For this review, take the finished solid that the model builds, in its own axes (mm). Face numbers are marked on the shaded views. A direction names the side the tool comes from. Give positions to 0.01 mm unless a question says otherwise; leave off trailing zeros. Loops run counter-clockwise (first coordinate to the right, second up) from the corner with the lowest first, then second, coordinate; pieces in that order, holes last. Notation, with made-up numbers: (85, -37) - (143, -37) arc R16 cw to (143, -32) - close; hole circle Ø2 at (5.25, 83). An arc over 180 degrees is marked (long way). Put each result on its own line as item: value. Start each with the question number.
from build123d import *

# Parameters (mm, degrees)
F0_W     = 40
F0_H     = 20
F1_DEPTH = 10
F2_DEPTH = 30
F3_DEPTH = 20
F4_W     = 10
F4_H     = 10
F5_DEPTH = 25


with BuildPart() as f1:
    # F0 (on Top) → F1 (new body)
    with BuildSketch(Plane.XY):
        Polygon((0, 40), (0, 20), (40, 20), (50, 20), (50, 40), align=None)
        with Locations((20, 10)):
            Rectangle(F0_W, F0_H)
        Polygon((40, 20), (40, 0), (60, 0), (60, 20), (50, 20), align=None)
    extrude(amount=-F1_DEPTH)

    # F0 (on Top) → F2 (join)
    with BuildSketch(Plane.XY):
        Polygon((0, 40), (0, 20), (40, 20), (50, 20), (50, 40), align=None)
    extrude(amount=F2_DEPTH)

    # F0 (on Top) → F3 (join)
    with BuildSketch(Plane.XY):
        Polygon((40, 20), (40, 0), (60, 0), (60, 20), (50, 20), align=None)
    extrude(amount=F3_DEPTH)

    # F4 (on face) → F5 (cut)
    with BuildSketch(Plane.YZ.offset(60)):
        with Locations((5, 5)):
            Rectangle(F4_W, F4_H)
    extrude(amount=-F5_DEPTH, mode=Mode.SUBTRACT)


solid = f1.part
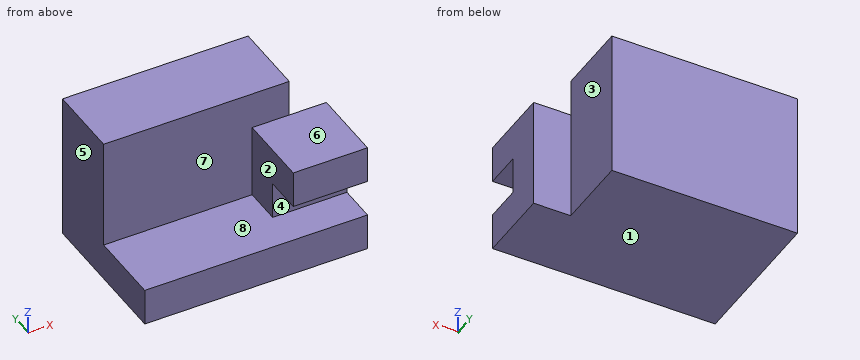
1) Machinability: for the marked faces 1, 2, 3, 4 and 5, which of the approach directions +Z, -Z, +X, -X, +Y, -Y give a long, thin tool a straight path to every point of the face, cutting with its end or side? Answer none if there is none.
2) Mouldability with a two-part tool opening along Z and no side actions: class the marked faces 6, 7 and 8 as released by +Z, released by -Z, zero draft, split by the parting line, or undercut.
3) Take a section at A-A on y = 6. State the section outline as (x, z) points.
4) Take a section at B-B on z = 2. State the section outline as (x, y) points, and give its area (3 significant figures).
5) Insertion check: P1, Ø10, axis at x = 48, y = 9.5, coming from the +Z side; P2, Ø16, axis at y = 9, z = 13, coming from the -X side; P3, Ø5, axis at x = 32.5, z = 22, coming from the -Y side. Each pin has a flat end and moves straight along its axis. Give the tip position at first contact, or say it passes through.
6) Take a section at C-C on x = 37. State the section outline as (y, z) points.
7) Wall thickness on probe 1 along Z at (x, y) = (42, 9.5); probe 2 along X at (y, z) = (25, 13.5); probe 3 along Y at (x, z) = (49.5, 22): over which ranges is each line inside the solid? List them lowest first.
8) Take a section at D-D on y = 35. State the section outline as (x, z) points.
Answers follow:
1. face 1: -Z, +X, -X, +Y, -Y
1. face 2: +Z, -X, -Y
1. face 3: +Z, -Z, +X, +Y
1. face 4: +X, -X, -Y
1. face 5: +Z, -Z, -X, +Y, -Y
2. face 6: released by +Z
2. face 7: zero draft
2. face 8: undercut
3. outline: (0, -10) - (60, -10) - (60, 0) - (0, 0) - close; (40, 10) - (60, 10) - (60, 20) - (40, 20) - close
4. outline: (0, 20) - (40, 20) - (40, 10) - (60, 10) - (60, 20) - (50, 20) - (50, 40) - (0, 40) - close
4. area: 1,200 mm2
5. P1: z = 20
5. P2: x = 40
5. P3: y = 20
6. outline: (0, -10) - (40, -10) - (40, 30) - (20, 30) - (20, 0) - (0, 0) - close
7. probe 1: -10 to 0, 10 to 20
7. probe 2: 0 to 50
7. probe 3: 20 to 40
8. outline: (0, -10) - (50, -10) - (50, 30) - (0, 30) - close
